```python
from build123d import *

# Parameters (mm, degrees)
EXTRUDE1_DEPTH = 0.2


with BuildPart() as part:
    # Sketch1 → Extrude1 (new body)
    with BuildSketch(Plane(origin=(0, 0, 0), x_dir=(1, 0, 0), z_dir=(0, 1, 0))):
        with BuildLine():
            Line((0, 10.5), (0.3, 7.5))
            Line((0.3, 7.5), (0.15, 0.734846923))
            ThreePointArc((0.15, 0.734846923), (0, -0.75), (-0.15, 0.734846923))
            Line((-0.15, 0.734846923), (-0.3, 7.5))
            Line((-0.3, 7.5), (0, 10.5))
        make_face()
    extrude(amount=EXTRUDE1_DEPTH)


solid = part.part
```
Geometry check sheet. Reference: the model listing, model coordinates, mm. Round coordinates to 2 decimals unless told otherwise and drop trailing zeros. Order: outer loops, then holes, each group sorted by start corner. A loop starts at its lowest first (then second) coordinate and runs counter-clockwise, first axis right, second up. Notation, with made-up numbers: M 34,72.25 L 72,72.25 A33 ccw 72,101.25 Z; hole C 9,59 d11. An arc over 180 degrees is marked long. Answer as CSV lines item,"result".
1) Sectioned sample at B-B on z = -2. Record the cut outline in (x, y).
Entries:
outline,"M -0.18,0 L 0.18,0 L 0.18,0.2 L -0.18,0.2 Z"
2) Thickness scan on probe 1 along Z at (x, y) = (-0.65, 0.1); probe 2 along X at (y, z) = (0.15, -6.75); probe 3 along Z at (x, y) = (-0.55, 0.1). Record the ranges inside material, lowest first. Write a range as [from, to].
Entries:
probe 1,"[-0.37, 0.37]"
probe 2,"[-0.28, 0.28]"
probe 3,"[-0.51, 0.51]"
3) Sectioned sample at C-C on x = 0.4. Record the cut outline in (y, z), and give its area (3 significant figures).
Entries:
outline,"M 0,-0.63 L 0.2,-0.63 L 0.2,0.63 L 0,0.63 Z"
area,"0.254 mm2"
4) Sectioned sample at A-A on y = 0.1. Record the cut outline in (x, z).
Entries:
outline,"M -0.3,-7.5 L 0,-10.5 L 0.3,-7.5 L 0.15,-0.73 A0.75 ccw long -0.15,-0.73 Z"
